Geometry: final body of the model. Coordinates: model frame, mm. Round coordinates to 2 decimals unless told otherwise and drop trailing zeros. Write each loop counter-clockwise with the first axis right and the second up, starting at its lowest first coordinate (ties: lowest second). Pieces come first, ordered by that corner, then holes. Notation, with made-up numbers: (-39, 81.25) - (7, 81.25) arc R14 ccw to (7, 95.25) - close; hole circle Ø8 at (-27, -17). An arc over 180 degrees is marked (long way). Use a Markdown table: item, result. Add a question column.
```python
from build123d import *

# Parameters (mm, degrees)
F0_W     = 136.290834
F0_H     = 85.74231
F1_DEPTH = 90.054186
F2_R     = 26.57018
F3_DEPTH = 175.134316
F4_R     = 36.09963


with BuildPart() as f1:
    # F0 (on Front) → F1 (new body)
    with BuildSketch(Plane.XZ):
        with Locations((14.668025, 0.729218)):
            Rectangle(F0_W, F0_H)
    extrude(amount=F1_DEPTH)

    # F2 (on face) → F3 (cut)
    with BuildSketch(Plane.XY.offset(43.600373)):
        with Locations((27.499106, -47.949214)):
            Circle(F2_R)
    extrude(amount=-F3_DEPTH, mode=Mode.SUBTRACT)

    # F4
    f4_edges = [f1.edges().sort_by_distance(p)[0] for p in [
        (82.813442, -90.054186, 0.729218),
    ]]
    fillet(f4_edges, radius=F4_R)


solid = f1.part
```
1) Draft query along Y for faces 1 (the flat face through (14, 0, 1)), 2 (the flat face through (-1, -44, 43.6)), 3 (the flat face through (-4, -90.054, 1)), 4 (the cylindrical face through (7.92, -29.99, 1.33)). Return one class per face: released by +Y, released by -Y, zero draft, split by the parting line, or undercut.
2) Material intervals for L1, parallel to X at y = -31.5, z = 36.5; L2, parallel to X at y = -67, z = 4.5; L3, parallel to Y at x = 19.5, z = 4.5, sorted ascending. Write a range as from..to.
3) Section C-C, the plane z = -21. Return the cut outline in (x, y), then the cut area to 3 significant figures.
4) Pin query (flat end, axial travel): P1, Ø1.5, axis at y = -71, z = 8.5, coming from the +X side. Return the tip coordinate at first contact, or that it passes through.
5) Section B-B, the plane y = -35.5. Return the cut outline in (x, z).
6) Section A-A, the plane x = 42.5. Return the cut outline in (y, z), then the cut area to 3 significant figures.
Output values:
| question | item | result |
|---|---|---|
| 1 | face 1 | released by +Y |
| 1 | face 2 | zero draft |
| 1 | face 3 | released by -Y |
| 1 | face 4 | undercut |
| 2 | L1 | x = -53.48..6.63, 48.37..82.81 |
| 2 | L2 | x = -53.48..8.98, 46.02..80.37 |
| 2 | L3 | y = -90.05..-73.29, -22.61..0 |
| 3 | outline | (-53.48, -90.05) - (46.71, -90.05) arc R36.1 ccw to (82.81, -53.95) - (82.81, 0) - (-53.48, 0) - close; hole circle Ø53.14 at (27.5, -47.95) |
| 3 | area | 9,780 mm^2 |
| 4 | P1 | stops at x = 78.93 |
| 5 | outline | (-53.48, -42.14) - (4.03, -42.14) - (4.03, 43.6) - (-53.48, 43.6) - close; (50.97, -42.14) - (82.81, -42.14) - (82.81, 43.6) - (50.97, 43.6) - close |
| 6 | outline | (-90.05, -42.14) - (-69.88, -42.14) - (-69.88, 43.6) - (-90.05, 43.6) - close; (-26.02, -42.14) - (0, -42.14) - (0, 43.6) - (-26.02, 43.6) - close |
| 6 | area | 3,960 mm^2 |
